```python
from build123d import *

# Parameters (mm, degrees)
F0_R     = 58.5
F1_DEPTH = 6.35


# Not quite as in the source:
# - a length typed as a fraction of an inch, garbled in the dataset ("3 / 203.2 mm" for 3/8 in), is restored


with BuildPart() as f1:
    # F0 (on Top) → F1 (new body)
    with BuildSketch(Plane.XY):
        with BuildLine():
            Line((67.5, 2.5), (73.4574706888, 2.5))
            ThreePointArc((73.4574706888, 2.5), (51.9723484172, 51.9723484172), (2.5, 73.4574706888))
            Line((2.5, 73.4574706888), (2.5, 67.5))
            ThreePointArc((2.5, 67.5), (0, 65), (-2.5, 67.5))
            Line((-2.5, 67.5), (-2.5, 73.4574706888))
            ThreePointArc((-2.5, 73.4574706888), (-51.9723484172, 51.9723484172), (-73.4574706888, 2.5))
            Line((-73.4574706888, 2.5), (-67.5, 2.5))
            ThreePointArc((-67.5, 2.5), (-65.732233047, 1.767766953), (-65, 0))
            ThreePointArc((-65, 0), (-65.732233047, -1.767766953), (-67.5, -2.5))
            Line((-67.5, -2.5), (-73.4574706888, -2.5))
            ThreePointArc((-73.4574706888, -2.5), (-51.9723484172, -51.9723484172), (-2.5, -73.4574706888))
            Line((-2.5, -73.4574706888), (-2.5, -67.5))
            ThreePointArc((-2.5, -67.5), (0, -65), (2.5, -67.5))
            Line((2.5, -67.5), (2.5, -73.4574706888))
            ThreePointArc((2.5, -73.4574706888), (51.9723484172, -51.9723484172), (73.4574706888, -2.5))
            Line((73.4574706888, -2.5), (67.5, -2.5))
            ThreePointArc((67.5, -2.5), (65, 0), (67.5, 2.5))
        make_face()
        Circle(F0_R, mode=Mode.SUBTRACT)
    extrude(amount=F1_DEPTH)


solid = f1.part
```
Here's how the part is built. I have some questions about the finished solid (model axes, mm). A direction names the side the tool comes from. Give positions to 0.01 mm unless a question says otherwise; leave off trailing zeros. Loops run counter-clockwise (first coordinate to the right, second up) from the corner with the lowest first, then second, coordinate; pieces in that order, holes last. Notation, with made-up numbers: (-12.75, 62.5) -> (30.25, 62.5) arc R9 cw to (30.25, 70.5) -> close; hole circle Ø1 at (-4, -19). An arc over 180 degrees is marked (long way). Use one line per item in the form item = value. Start each with the question number.
1) Thinking about a two-plate mould opening in Y: for faces 1 (the face through (-51.42, 52.52, 3.13)), 2 (the face through (-2.5, 70, 3)), 3 (the face through (71, -2.5, 3)), which applies, +Y half, -Y half, draft (parallel to the pull), parting line (faces both ways), or undercut?
2) Imagine slicing it at B-B (z = 1.5). Please give me the cut outline in (x, y).
3) Which directions (+Z, -Z, +X, -X, +Y, -Y) give clear straight access to the entire face, cutting with the end or side of a thin tool? Please do faces 4 (the face through (-2.5, -71, 3)), 5 (the face through (2.5, 71, 3)), 6 (the face through (70, 2.5, 3)), 7 (the face through (-71, 2.5, 3)).
4) Imagine slicing it at A-A (x = 0). Please give me the cut outline in (y, z), then the cut area to 4 significant figures.
5) Please list where these lines run through material, in increasing order: line 1 along Y through (x, z) = (0, 1.5); line 2 along X through (y, z) = (18, 2); line 3 along Y through (x, z) = (31, 3.5).
6) Imagine slicing it at D-D (x = 62). Please give me the cut outline in (y, z).
7) For P1, Ø3, axis at y = -69.5, z = 4, coming from the -X side; P2, Ø1, axis at x = -27, z = 4, coming from the -Y side; P3, Ø2, axis at y = -41, z = 2, coming from the +X side, each with a flat end and sliding along its axis, tell me the tip position at first contact or that it passes through.
8) Imagine slicing it at C-C (y = 49). Please give me the cut outline in (x, z), then the cut area to 3 significant figures.
Check values:
q1.face_1 = +Y half
q1.face_2 = draft
q1.face_3 = undercut
q2.outline = (-73.46, -2.5) arc R73.5 ccw to (-2.5, -73.46) -> (-2.5, -67.5) arc R2.5 cw to (2.5, -67.5) -> (2.5, -73.46) arc R73.5 ccw to (73.46, -2.5) -> (67.5, -2.5) arc R2.5 cw to (67.5, 2.5) -> (73.46, 2.5) arc R73.5 ccw to (2.5, 73.46) -> (2.5, 67.5) arc R2.5 cw to (-2.5, 67.5) -> (-2.5, 73.46) arc R73.5 ccw to (-73.46, 2.5) -> (-67.5, 2.5) arc R2.5 cw to (-67.5, -2.5) -> close; hole circle Ø117 at (0, 0)
q3.face_4 = +Z, -Z, -Y
q3.face_5 = +Z, -Z, +Y
q3.face_6 = +Z, -Z, +X
q3.face_7 = +Z, -Z, -X
q4.outline = (-65, 0) -> (-58.5, 0) -> (-58.5, 6.35) -> (-65, 6.35) -> close; (58.5, 0) -> (65, 0) -> (65, 6.35) -> (58.5, 6.35) -> close
q4.area = 82.55 mm^2
q5.line_1 = -65 to -58.5, 58.5 to 65
q5.line_2 = -71.26 to -55.66, 55.66 to 71.26
q5.line_3 = -66.64 to -49.61, 49.61 to 66.64
q6.outline = (-39.47, 0) -> (39.47, 0) -> (39.47, 6.35) -> (-39.47, 6.35) -> close
q7.P1 = -27.9
q7.P2 = -68.56
q7.P3 = 61.66
q8.outline = (-54.78, 0) -> (-31.96, 0) -> (-31.96, 6.35) -> (-54.78, 6.35) -> close; (31.96, 0) -> (54.78, 0) -> (54.78, 6.35) -> (31.96, 6.35) -> close
q8.area = 290 mm^2
